Geometry: final body of the model. Coordinates: model frame, mm. Round coordinates to 2 decimals unless told otherwise and drop trailing zeros. Write each loop counter-clockwise with the first axis right and the second up, starting at its lowest first coordinate (ties: lowest second). Pieces come first, ordered by that corner, then holes. Notation, with made-up numbers: (62, -9) - (69, -9) arc R24 ccw to (69, 3) - close; hole circle Ø1 at (83.5, 50.5). An arc over 180 degrees is marked (long way). Use a Markdown table: item, result. Add a question column.
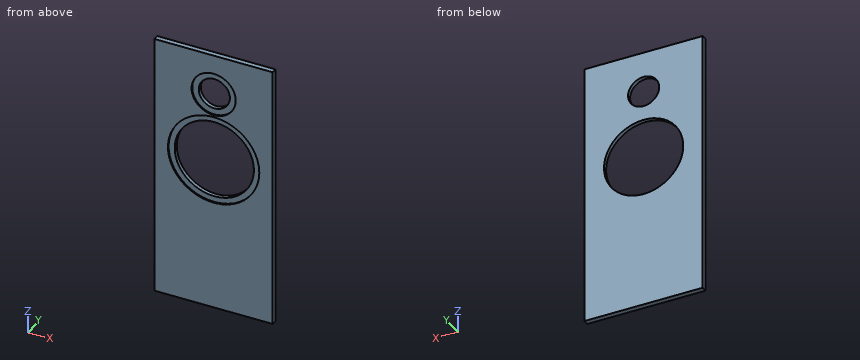
```python
from build123d import *

# Parameters (mm, degrees)
F0_W     = 279.4
F0_H     = 635
F1_DEPTH = 12.7
F2_R     = 52.197
F2_R_2   = 107.95
F3_DEPTH = 3.175
F4_R     = 36.83
F4_R_2   = 93.6625
F5_DEPTH = 12.701


with BuildPart() as f1:
    # F0 (on Front) → F1 (new body)
    with BuildSketch(Plane.XZ):
        with Locations((139.7, 317.5)):
            Rectangle(F0_W, F0_H)
    extrude(amount=F1_DEPTH)

    # F2 (on face) → F3 (cut)
    with BuildSketch(Plane.XZ.offset(12.7)):
        with Locations((139.7, 537.082911)):
            Circle(F2_R)
        with Locations((139.7, 371.982911)):
            Circle(F2_R_2)
    extrude(amount=-F3_DEPTH, mode=Mode.SUBTRACT)

    # F4 (on face) → F5 (cut, through all)
    with BuildSketch(Plane.XZ.offset(12.7)):
        with Locations((139.7, 537.082911)):
            Circle(F4_R)
        with Locations((139.7, 371.982911)):
            Circle(F4_R_2)
    extrude(amount=-F5_DEPTH, mode=Mode.SUBTRACT)


solid = f1.part
```
1) Section D-D, the plane z = 359.5. Return the cut outline in (x, y) (3 decimals), then the cut area to 3 significant figures.
2) Pin query (flat end, axial travel): P1, Ø12, axis at x = 54.5, z = 421.5, coming from the -Y side (3 decimals). Return the tip coordinate at first contact, or that it passes through.
3) Section A-A, the plane x = 139.7. Return the cut outline in (y, z) (3 decimals).
4) Material intervals for L1, parallel to Z at x = 139.7, y = -5.25; L2, parallel to Z at x = 139.7, y = -10.65; L3, parallel to X at y = -9.25, z = 369.5, sorted ascending. Write a range as from..to.
5) Section B-B, the plane z = 518.5. Return the cut outline in (x, y) (3 decimals).
6) Section C-C, the plane y = -4.5. Return the cut outline in (x, z) (1 decimal), then the cut area to 3 significant figures.
Output values:
| question | item | result |
|---|---|---|
| 1 | outline | (0, -12.7) - (32.474, -12.7) - (32.474, -9.525) - (46.873, -9.525) - (46.873, 0) - (0, 0) - close; (232.527, -9.525) - (246.926, -9.525) - (246.926, -12.7) - (279.4, -12.7) - (279.4, 0) - (232.527, 0) - close |
| 1 | area | 1,100 mm^2 |
| 2 | P1 | stops at y = -9.525 |
| 3 | outline | (-12.7, 0) - (0, 0) - (0, 278.32) - (-9.525, 278.32) - (-9.525, 264.033) - (-12.7, 264.033) - close; (-12.7, 479.933) - (-9.525, 479.933) - (-9.525, 465.645) - (0, 465.645) - (0, 500.253) - (-9.525, 500.253) - (-9.525, 484.886) - (-12.7, 484.886) - close; (-12.7, 589.28) - (-9.525, 589.28) - (-9.525, 573.913) - (0, 573.913) - (0, 635) - (-12.7, 635) - close |
| 4 | L1 | z = 0..278.32, 465.65..500.25, 573.91..635 |
| 4 | L2 | z = 0..264.03, 479.93..484.89, 589.28..635 |
| 4 | L3 | x = 0..46.07, 233.33..279.4 |
| 5 | outline | (0, -12.7) - (90.923, -12.7) - (90.923, -9.525) - (107.902, -9.525) - (107.902, 0) - (0, 0) - close; (171.498, -9.525) - (188.477, -9.525) - (188.477, -12.7) - (279.4, -12.7) - (279.4, 0) - (171.498, 0) - close |
| 6 | outline | (0, 0) - (279.4, 0) - (279.4, 635) - (0, 635) - close; hole circle Ø187.3 at (139.7, 372); hole circle Ø73.7 at (139.7, 537.1) |
| 6 | area | 146,000 mm^2 |
